Part print with two shaded views. Sizes in mm from the minimum x, y, z corner. A direction names the side the tool comes from. Round coordinates to 2 decimals unless told otherwise and drop trailing zeros. Order: outer loops, then holes, each group sorted by start corner. A loop starts at its lowest first (then second) coordinate and runs counter-clockwise, first axis right, second up. Notation, with made-up numbers: M 53,56.5 L 84,56.5 A7 cw 84,61.5 Z; hole C 72.25,7 d3. An arc over 180 degrees is marked long. One line per question, with ' | ' between items.
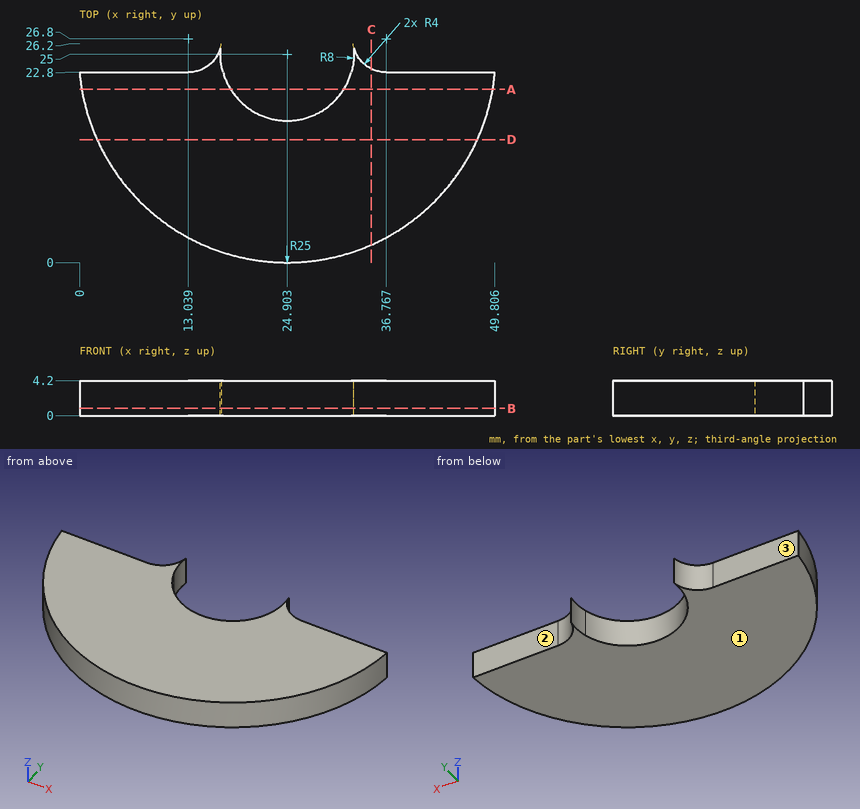
1) Saw through at B-B (z = 0.85). List the corners of the cut face in (x, y) (1 decimal).
The answers:
outline: M 0,22.8 A25 ccw 49.8,22.8 L 36.8,22.8 A4 cw 32.8,26.2 A8 cw long 17,26.2 A4 cw 13,22.8 Z
2) Probe line 1 (X direction, y = 23.25, z = 2.45) (1 decimal); line 2 (Y direction, x = 6, z = 3.55); line 3 (Y direction, x = 26.5, z = 1.85). List the from-to ranges inside material, lowest first. Write a range as [from, to].
The answers:
line 1: x = [14.9, 17.1], [32.7, 34.9] | line 2: y = [8.64, 22.8] | line 3: y = [0.05, 17.16]
3) Saw through at A-A (y = 20.75). List the corners of the cut face in (x, z) (1 decimal), plus the area to 3 significant figures.
The answers:
outline: M 0.3,0 L 18.1,0 L 18.1,4.2 L 0.3,4.2 Z; M 31.7,0 L 49.5,0 L 49.5,4.2 L 31.7,4.2 Z | area: 150 mm²
4) Drop a flat-ended pin along its axis: pin 1 (1.3 mm diameter, centred on x = 44.5, z = 2.5, fed in from +Y). Give the stop position or say it passes through.
The answers:
pin 1: stops at y = 22.8
5) Saw through at C-C (x = 35). List the corners of the cut face in (y, z).
The answers:
outline: M 2.13,0 L 23.21,0 L 23.21,4.2 L 2.13,4.2 Z
6) Which spindle directions (+Z, -Z, +X, -X, +Y, -Y) get a long thin tool onto all of the face, cutting with end or side? Do the marked faces 1, 2 and 3. Say none if no direction does.
The answers:
face 1: -Z, +X, -X, +Y, -Y | face 2: +Z, -Z, +X, +Y | face 3: +Z, -Z, -X, +Y
7) Saw through at D-D (y = 14.75). List the corners of the cut face in (x, z) (1 decimal).
The answers:
outline: M 2.1,0 L 47.7,0 L 47.7,4.2 L 2.1,4.2 Z
